from build123d import *

# Parameters (mm, degrees)
BOSS_EXTRUDE1_DEPTH = 2.5
SKETCH6_W           = 70
SKETCH6_H           = 2.5
SKETCH6_W_2         = 2.5
SKETCH6_H_2         = 30
CUT_EXTRUDE3_DEPTH  = 3.5
SKETCH7_R           = 8
CUT_EXTRUDE4_DEPTH  = 3.5


with BuildPart() as part:
    # Sketch2 → Boss-Extrude1 (new body)
    with BuildSketch(Plane(origin=(0, 0, 0), x_dir=(1, 0, 0), z_dir=(0, 1, 0))):
        Polygon((0, 0), (170, 0), (170, 135), (145.104076401, 195.104076401), (85, 220), (24.895923599, 195.104076401), (0, 135), align=None)
    extrude(amount=BOSS_EXTRUDE1_DEPTH)

    # Sketch6 → Cut-Extrude3 (cut, through all)
    with BuildSketch(Plane(origin=(0, 2.5, 0), x_dir=(1, 0, 0), z_dir=(0, 1, 0))):
        with Locations((85, 1.25)):
            Rectangle(SKETCH6_W, SKETCH6_H)
        Polygon((170, 0), (170, 20), (167.5, 20), (167.5, 2.5), (150, 2.5), (150, 0), align=None)
        Polygon((145.104076401, 195.104076401), (130.289174832, 201.240609556), (129.332466251, 198.930910725), (143.190659239, 193.190659239), (167.5, 134.502719082), (167.5, 110), (170, 110), (170, 135), align=None)
        with Locations((168.75, 65)):
            Rectangle(SKETCH6_W_2, SKETCH6_H_2)
        Polygon((101.616080276, 210.411413695), (102.572788857, 212.721112527), (85, 220), (67.427211143, 212.721112527), (68.383919724, 210.411413695), (85, 217.294019499), align=None)
        Polygon((0, 110), (0, 135), (24.895923599, 195.104076401), (39.710825168, 201.240609556), (40.667533749, 198.930910725), (26.809340761, 193.190659239), (2.5, 134.502719082), (2.5, 110), align=None)
        with Locations((1.25, 65)):
            Rectangle(SKETCH6_W_2, SKETCH6_H_2)
        Polygon((20, 0), (0, 0), (0, 20), (2.5, 20), (2.5, 2.5), (20, 2.5), align=None)
    extrude(amount=-CUT_EXTRUDE3_DEPTH, mode=Mode.SUBTRACT)

    # Sketch7 → Cut-Extrude4 (cut, through all)
    with BuildSketch(Plane(origin=(0, 2.5, 0), x_dir=(1, 0, 0), z_dir=(0, 1, 0))):
        with Locations((72, 187.294019499)):
            Circle(SKETCH7_R)
        with Locations((98, 187.294019499)):
            Circle(SKETCH7_R)
    extrude(amount=-CUT_EXTRUDE4_DEPTH, mode=Mode.SUBTRACT)


solid = part.part
Part model, mm, in its own coordinate system. A direction names the side the tool comes from. Round coordinates to 2 decimals unless told otherwise and drop trailing zeros. Write each loop counter-clockwise with the first axis right and the second up, starting at its lowest first coordinate (ties: lowest second). Pieces come first, ordered by that corner, then holes. Notation, with made-up numbers: (48, -11) - (102, -11) arc R30 cw to (102, 21) - close; hole circle Ø9 at (5, 71.25). An arc over 180 degrees is marked (long way). Use CSV: the item, a comma, the result in double quotes.
Item 1: Slice it at B-B, the plane z = -59. Write the cut outline in (x, y), then the cut area to 4 significant figures.
Results list:
outline,"(2.5, 0) - (167.5, 0) - (167.5, 2.5) - (2.5, 2.5) - close"
area,"412.5 mm²"
Item 2: Pull direction X, two halves, no side cores. Call faces 1 (the flat face through (116.625, 1.232, -206.9)), 2 (the flat face through (76.576, 1.268, -213.805)), 3 (the flat face through (33.835, 1.268, -196.101)): pulls with the +X half, pulls with the -X half, needs draft (parallel to the pull), parting line crosses it, or undercut.
Results list:
face 1,"pulls with the +X half"
face 2,"undercut"
face 3,"pulls with the -X half"
Item 3: Flat gauge pins, fed straight in: P1, Ø1.5, axis at x = 19.5, y = 0.5, coming from the -Z side (3 decimals); P2, Ø1.2, axis at x = 159, y = 1.5, coming from the +Z side; P3, Ø0.8, axis at y = 1.5, z = -8.5, coming from the -X side; P4, Ø14.5, axis at x = 72, z = -187.29, coming from the -Y side. Where does each tip first touch, or does it go through?
Results list:
P1,"stops at z = -177.355"
P2,"stops at z = -2.5"
P3,"stops at x = 2.5"
P4,"passes through"
Item 4: Tool access for faces 4 (the flat face through (93.19, 1.27, -213.9)), 5 (the flat face through (84, 0, -86)): list every direction of +Z, -Z, +X, -X, +Y, -Y with a clear straight run to the whole face (end or side of a thin tool).
Results list:
face 4,"-Z, +Y, -Y"
face 5,"+Z, -Z, +X, -X, -Y"
Item 5: Wall check: L1, parallel to X at y = 1.65, z = -185; L2, parallel to X at y = 1.6, z = -185.5; L3, parallel to X at y = 0.75, z = -123. Give the ranges that are in metal, low to high.
Results list:
L1,"x = 23.42 to 64.34, 79.66 to 90.34, 105.66 to 146.58"
L2,"x = 23.62 to 64.2, 79.8 to 90.2, 105.8 to 146.38"
L3,"x = 2.5 to 167.5"
Item 6: Slice it at D-D, the plane x = 157.5. Write the cut outline in (y, z).
Results list:
outline,"(0, -158.64) - (2.5, -158.64) - (2.5, -2.5) - (0, -2.5) - close"
Item 7: Slice it at C-C, the plane y = 0.5. Count the separate pieces of the cut face and the enclosed holes in it, then the cut area to 3 significant figures.
Results list:
separate pieces,"1"
enclosed holes,"2"
area,"31,600 mm²"
Item 8: Slice it at A-A, the plane x = 98. Write the cut outline in (y, z).
Results list:
outline,"(0, -211.91) - (2.5, -211.91) - (2.5, -195.29) - (0, -195.29) - close; (0, -179.29) - (2.5, -179.29) - (2.5, -2.5) - (0, -2.5) - close"
